Check sheet for the modelled part. Datum: model origin and axes. Units: mm. Coordinates: 2 decimals unless noted, no trailing zeros. Loops run counter-clockwise (first coordinate to the right, second up) from the corner with the lowest first, then second, coordinate; pieces in that order, holes last.
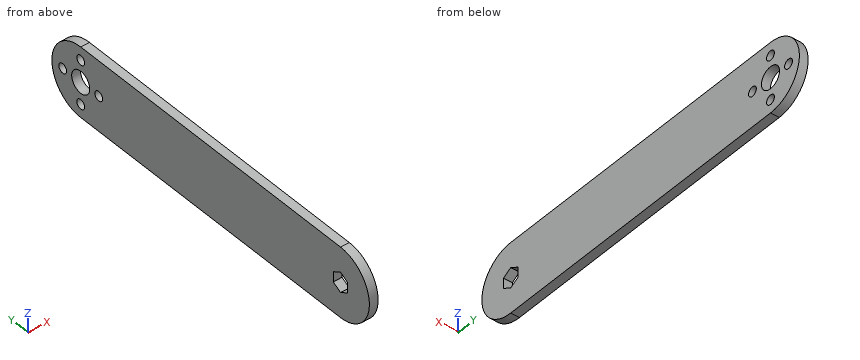
```python
from build123d import *

# Parameters (mm, degrees)
SKETCH1_R           = 7.9375
SKETCH1_R_2         = 3.429
BOSS_EXTRUDE1_DEPTH = 6.35


with BuildPart() as part:
    # Sketch1 → Boss-Extrude1 (new body)
    with BuildSketch(Plane(origin=(0, 0, 0), x_dir=(0, 0, -1), z_dir=(1, 0, 0))):
        with BuildLine():
            Line((-25.4, 228.6), (-25.4, 0))
            ThreePointArc((-25.4, 0), (0, -25.4), (25.4, 0))
            Line((25.4, 0), (25.4, 228.6))
            ThreePointArc((25.4, 228.6), (0, 254), (-25.4, 228.6))
        make_face()
        with Locations((0, 228.6)):
            Circle(SKETCH1_R, mode=Mode.SUBTRACT)
        with Locations((0, 212.725)):
            Circle(SKETCH1_R_2, mode=Mode.SUBTRACT)
        with Locations((-15.875, 228.6)):
            Circle(SKETCH1_R_2, mode=Mode.SUBTRACT)
        with Locations((0, 244.475)):
            Circle(SKETCH1_R_2, mode=Mode.SUBTRACT)
        with Locations((15.875, 228.6)):
            Circle(SKETCH1_R_2, mode=Mode.SUBTRACT)
        Polygon((7.332348419, 0), (3.666174209, 6.35), (-3.666174209, 6.35), (-7.332348419, 0), (-3.666174209, -6.35), (3.666174209, -6.35), align=None, mode=Mode.SUBTRACT)
    extrude(amount=BOSS_EXTRUDE1_DEPTH)


solid = part.part
```
1) Scan lines: line 1 (Y direction, x = 5, z = 0); line 2 (Y direction, x = 5.75, z = -2.5); line 3 (Y direction, x = 0.5, z = -15.5). Record each from-to range of solid material in increasing order.
Answer sheet:
line 1: y = -25.4 to -6.35, 6.35 to 209.3, 216.15 to 220.66, 236.54 to 241.05, 247.9 to 254
line 2: y = -25.28 to -6.35, 6.35 to 210.38, 215.07 to 221.07, 236.13 to 242.13, 246.82 to 253.88
line 3: y = -20.12 to 225.19, 232.01 to 248.72
2) Section check B-B on z = -16. Enter the section's corners in (x, y).
Answer sheet:
outline: (0, -19.73) - (6.35, -19.73) - (6.35, 225.17) - (0, 225.17) - close; (0, 232.03) - (6.35, 232.03) - (6.35, 248.33) - (0, 248.33) - close
3) Section check C-C on x = 4.75. Give the number of separate pieces and of enclosed holes in the cut face, plus the area to 3 significant figures.
Answer sheet:
separate pieces: 1
enclosed holes: 6
area: 13,200 mm2
4) Depth check by flat-ended pin: pin 1 (1.9 mm diameter, centred on x = 3, z = -0.5, fed in from +Y); pin 2 (3 mm diameter, centred on x = 2, z = 13, fed in from -Y); pin 3 (1 mm diameter, centred on x = 2.5, z = 9, fed in from -Y). Enter the tip coordinate at first touch or a pass-through.
Answer sheet:
pin 1: stops at y = 254
pin 2: stops at y = -22.65
pin 3: stops at y = -23.94
5) Section check A-A on z = 0. Enter the section's corners in (x, y), plus the area to 3 significant figures.
Answer sheet:
outline: (0, -25.4) - (6.35, -25.4) - (6.35, -6.35) - (0, -6.35) - close; (0, 6.35) - (6.35, 6.35) - (6.35, 209.3) - (0, 209.3) - close; (0, 216.15) - (6.35, 216.15) - (6.35, 220.66) - (0, 220.66) - close; (0, 236.54) - (6.35, 236.54) - (6.35, 241.05) - (0, 241.05) - close; (0, 247.9) - (6.35, 247.9) - (6.35, 254) - (0, 254) - close
area: 1,510 mm2
